from build123d import *

# Parameters (mm, degrees)
F1_DEPTH       = 34.925
F3_D           = 8.8
F3_DEPTH       = 20.6375
F3_CBORE_D     = 14.25
F3_CBORE_DEPTH = 8
F3_TIP         = 2.6437867237
F5_D           = 6.8
F5_DEPTH       = 20.6375
F5_TIP         = 2.0429261047
F6_R           = 3.175
F7_SIZE        = 0.762
F9_D           = 6.8


# Not quite as in the source:
# - ends of sketch curves that miss each other by under 0.0002 mm in the source are joined


with BuildPart() as f1:
    # F0 (on Top) → F1 (new body, symmetric)
    with BuildSketch(Plane.XY):
        with BuildLine():
            Line((-30.1270424985, 1.5875), (-30.1270424985, -31.75))
            Line((-30.1270424985, -31.75), (-15.6690329313, -31.75))
            Line((-15.6690329313, -31.75), (-10.9754424985, -31.75))
            Line((-10.9754424985, -31.75), (-10.9754424985, -12.6142650107))
            ThreePointArc((-10.9754424985, -12.6142650107), (-19.4991930627, -7.8326866028), (-22.1026331175, 1.5875))
            ThreePointArc((-22.1026331175, 1.5875), (-0.5628331886, 9.0209179793), (-7.8004424985, -12.585462914))
            Line((-7.8004424985, -12.585462914), (-7.8004424985, -31.75))
            Line((-7.8004424985, -31.75), (15.8469575015, -31.75))
            Line((15.8469575015, -31.75), (15.8977575015, 0))
            Line((15.8977575015, 0), (34.9477575015, 0))
            Line((34.9477575015, 0), (34.9477575015, 19.05))
            Line((34.9477575015, 19.05), (-30.1270424985, 19.05))
            Line((-30.1270424985, 19.05), (-30.1270424985, 1.5875))
        make_face()
    extrude(amount=F1_DEPTH, both=True)

    # F3
    with Locations(Plane(origin=(-30.1270424985, 0, 0), x_dir=(0, -1, 0), z_dir=(-1, 0, 0))):
        with Locations((23.8125, 25.4), (23.8125, -25.4)):
            CounterBoreHole(F3_D / 2, F3_CBORE_D / 2, F3_CBORE_DEPTH, depth=F3_DEPTH)
            with Locations((0, 0, -(F3_DEPTH + F3_TIP / 2))):  # 118° drill point
                Cone(0, F3_D / 2, F3_TIP, mode=Mode.SUBTRACT)

    # F5
    with Locations(Plane(origin=(-30.1270424985, 0, 0), x_dir=(0, -1, 0), z_dir=(-1, 0, 0))):
        with Locations((24.2870002985, 0)):
            Hole(F5_D / 2, depth=F5_DEPTH)
            with Locations((0, 0, -(F5_DEPTH + F5_TIP / 2))):  # 118° drill point
                Cone(0, F5_D / 2, F5_TIP, mode=Mode.SUBTRACT)

    # F6
    f6_edges = [f1.edges().sort_by_distance(p)[0] for p in [
        (15.897758, 0, 0),
    ]]
    fillet(f6_edges, radius=F6_R)

    # F7
    f7_edges = [f1.edges().sort_by_distance(p)[0] for p in [
        (-9.617446, 12.699477, 34.925),
        (-9.617446, 12.699477, -34.925),
    ]]
    chamfer(f7_edges, length=F7_SIZE)

    # F9 (through all)
    with Locations(Plane(origin=(15.8977168033, -0.0254363469, 0), x_dir=(0.001599998, 0.99999872, 0), z_dir=(0.99999872, -0.001599998, 0))):
        with Locations((-23.7871042605, 25.4), (-23.7871042605, -25.4)):
            Hole(F9_D / 2)


solid = f1.part
Work out the finished part from the listing and answer in its coordinate system (mm). A direction names the side the tool comes from. Give positions to 0.01 mm unless a question says otherwise; leave off trailing zeros. Write each loop counter-clockwise with the first axis right and the second up, starting at its lowest first coordinate (ties: lowest second). Pieces come first, ordered by that corner, then holes.
Q1. The part is cut by section D-D on z = 1.5. Give the vertices of the cut face in (x, y) (3 decimals).
Answer:
outline: (-30.127, -31.75) - (-10.975, -31.75) - (-10.975, -27.338) - (-30.127, -27.338) - close; (-30.127, -21.236) - (-10.975, -21.236) - (-10.975, -12.614) arc R12.7 cw (long way) to (-7.8, -12.585) - (-7.8, -31.75) - (15.847, -31.75) - (15.893, -3.17) arc R3.175 cw to (19.068, 0) - (34.948, 0) - (34.948, 19.05) - (-30.127, 19.05) - close
Q2. The part is cut by section B-B on x = -1. State how many separate pieces and enclosed holes the cut face has, and give its area (3 significant figures).
Answer:
separate pieces: 2
enclosed holes: 2
area: 2,160 mm2
Q3. A tool of negligible diameter and unlimited length cuts with its end or side. For faces 1 (the face through (-26.183, -22.268, 18.444)), 2 (the face through (3, 19.05, 0)), 3 (the face through (-21, -31.75, 0)), 4 (the face through (27, 0, 0)), 5 (the face through (-7.8, -22, 0)), from which of +Z, -Z, +X, -X, +Y, -Y can it reach the whole face along a straight path? Write none if from no direction.
Answer:
face 1: -X
face 2: +Z, -Z, +X, -X, +Y
face 3: +Z, -Z, +X, -X, -Y
face 4: +Z, -Z, +X, -Y
face 5: +Z, -Z, -Y
Q4. Given pin 1 (7 mm diameter, centred on y = -24, z = -26, fed in from -X); pin 2 (11 mm diameter, centred on y = -24.287, z = 0, fed in from +X); pin 3 (12.5 mm diameter, centred on x = 26.5, z = -6, fed in from -Y); pin 4 (10 mm diameter, centred on y = -4, z = 17, fed in from +X), each flat-ended and moving along its own axis, determine where each tip first touches the part or whether it passes through.
Answer:
pin 1: stops at x = -7.8
pin 2: stops at x = 15.87
pin 3: stops at y = 0
pin 4: stops at x = 34.95
Q5. The part is cut by section A-A on z = 16.5. Give the vertices of the cut face in (x, y) (3 decimals), and give its area (3 significant figures).
Answer:
outline: (-30.127, -31.75) - (-10.975, -31.75) - (-10.975, -12.614) arc R12.7 cw (long way) to (-7.8, -12.585) - (-7.8, -31.75) - (15.847, -31.75) - (15.893, -3.17) arc R3.175 cw to (19.068, 0) - (34.948, 0) - (34.948, 19.05) - (-30.127, 19.05) - close
area: 2,140 mm2
Q6. For a pull along X with two mould halves and no side action, classify faces 6 (the face through (-10.153, 12.683, 0.478)), 7 (the face through (-16.473, -24.766, 21.105)) as released by +X, released by -X, zero draft, split by the parting line, or undercut.
Answer:
face 6: undercut
face 7: zero draft
Q7. Straight lines are drawn through the part: L1, parallel to Z at x = -1.5, y = -24 (3 decimals); L2, parallel to X at y = -19.5, z = -20; L3, parallel to Z at x = -27, y = -23.5 (3 decimals). For each, find the intervals that lie inside material, in ascending order.
Answer:
L1: z = -34.925 to -28.793, -22.007 to 22.007, 28.793 to 34.925
L2: x = -22.13 to -10.98, -7.8 to 15.87
L3: z = -34.925 to -32.518, -18.282 to -3.308, 3.308 to 18.282, 32.518 to 34.925
